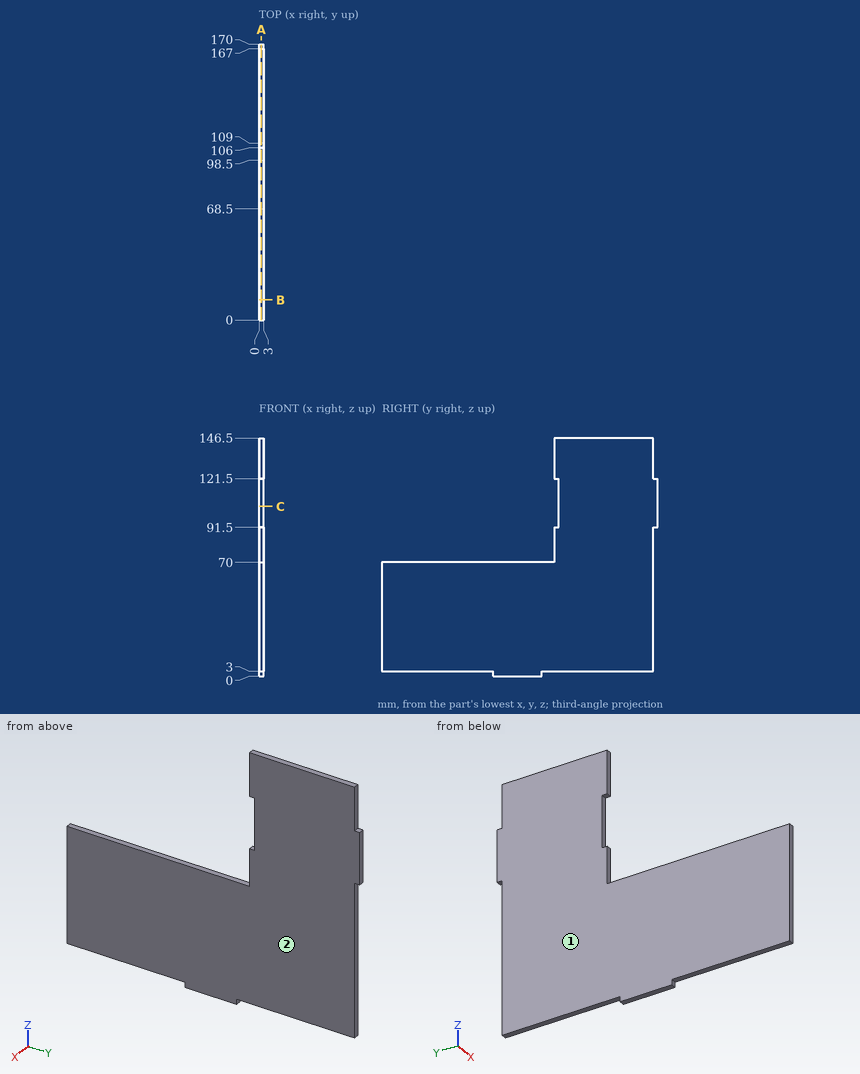
Geometry: see drawing. Coordinates: mm, zero at the bounding-box minimum. Give positions to 0.01 mm unless a question says otherwise; leave off trailing zeros. Loops run counter-clockwise (first coordinate to the right, second up) from the corner with the lowest first, then second, coordinate; pieces in that order, holes last. Notation, with made-up numbers: (-15, -36.5) -> (-6, -36.5) arc R12 cw to (-6, -18.5) -> close; hole circle Ø6 at (-5, 35). An arc over 180 degrees is marked (long way). Use one line per item in the form item = value.
Item 1: Section query B-B on y = 12.5. Output: boundary loops of the cut face in (x, z), and give its area (3 significant figures).
A:
outline = (0, 3) -> (3, 3) -> (3, 70) -> (0, 70) -> close
area = 201 mm^2
Item 2: Draft query along X for the marked faces 1 and 2. Return one class per face: pulls with the +X half, pulls with the -X half, needs draft (parallel to the pull), parting line crosses it, or undercut.
A:
face_1 = pulls with the -X half
face_2 = pulls with the +X half
Item 3: Section query C-C on z = 104.5. Output: boundary loops of the cut face in (x, y).
A:
outline = (0, 109) -> (3, 109) -> (3, 170) -> (0, 170) -> close
Item 4: Pin query (flat end, axial travel): P1, Ø0.9, axis at x = 2, z = 1.5, coming from the +Y side; P2, Ø0.9, axis at x = 1, y = 169, coming from the +Z side; P3, Ø1.5, axis at x = 2, z = 105, coming from the -Y side. Return the tip coordinate at first contact, or that it passes through.
A:
P1 = 98.5
P2 = 121.5
P3 = 109
Item 5: Line query: probe 1 along Y at (x, z) = (0.3, 57); probe 2 along Z at (x, y) = (0.35, 77); probe 3 along Y at (x, z) = (2.85, 129.5). Output: solid intervals per line, ascending.
A:
probe_1 = 0 to 167
probe_2 = 0 to 70
probe_3 = 106 to 167
Item 6: Section query A-A on x = 1.5. Output: boundary loops of the cut face in (y, z), and give its area (3 significant figures).
A:
outline = (0, 3) -> (68.5, 3) -> (68.5, 0) -> (98.5, 0) -> (98.5, 3) -> (167, 3) -> (167, 91.5) -> (170, 91.5) -> (170, 121.5) -> (167, 121.5) -> (167, 146.5) -> (106, 146.5) -> (106, 121.5) -> (109, 121.5) -> (109, 91.5) -> (106, 91.5) -> (106, 70) -> (0, 70) -> close
area = 15,900 mm^2
